from build123d import *

# Parameters (mm, degrees)
F0_W     = 152.4
F0_H     = 25.4
F1_DEPTH = 50.8
F2_D     = 4.2
F2_DEPTH = 18
F2_TIP   = 1.2618073
F3_D     = 5
F3_DEPTH = 20
F3_TIP   = 1.5021515476
F4_D     = 6.8
F4_DEPTH = 25
F4_TIP   = 2.0429261047
F5_D     = 8.5
F5_DEPTH = 25
F5_TIP   = 2.5536576309
F6_D     = 10.3
F6_DEPTH = 40
F6_TIP   = 3.094432188
F7_R     = 2


with BuildPart() as f1:
    # F0 (on Top) → F1 (new body)
    with BuildSketch(Plane.XY):
        with Locations((22.0912756948, 0)):
            Rectangle(F0_W, F0_H)
    extrude(amount=-F1_DEPTH)

    # F2
    with Locations(Plane.XY):
        with Locations((-28.7087243052, 0)):
            Hole(F2_D / 2, depth=F2_DEPTH)
            with Locations((0, 0, -(F2_DEPTH + F2_TIP / 2))):  # 118° drill point
                Cone(0, F2_D / 2, F2_TIP, mode=Mode.SUBTRACT)

    # F3
    with Locations(Plane.XY):
        with Locations((-3.3087243052, 0)):
            Hole(F3_D / 2, depth=F3_DEPTH)
            with Locations((0, 0, -(F3_DEPTH + F3_TIP / 2))):  # 118° drill point
                Cone(0, F3_D / 2, F3_TIP, mode=Mode.SUBTRACT)

    # F4
    with Locations(Plane.XY):
        with Locations((22.0912756948, 0)):
            Hole(F4_D / 2, depth=F4_DEPTH)
            with Locations((0, 0, -(F4_DEPTH + F4_TIP / 2))):  # 118° drill point
                Cone(0, F4_D / 2, F4_TIP, mode=Mode.SUBTRACT)

    # F5
    with Locations(Plane.XY):
        with Locations((47.4912756948, 0)):
            Hole(F5_D / 2, depth=F5_DEPTH)
            with Locations((0, 0, -(F5_DEPTH + F5_TIP / 2))):  # 118° drill point
                Cone(0, F5_D / 2, F5_TIP, mode=Mode.SUBTRACT)

    # F6
    with Locations(Plane.XY):
        with Locations((72.8912756948, 0)):
            Hole(F6_D / 2, depth=F6_DEPTH)
            with Locations((0, 0, -(F6_DEPTH + F6_TIP / 2))):  # 118° drill point
                Cone(0, F6_D / 2, F6_TIP, mode=Mode.SUBTRACT)

    # F7
    f7_edges = [f1.edges().sort_by_distance(p)[0] for p in [
        (22.091276, -12.7, 0),
        (98.291276, 0, 0),
        (22.091276, 12.7, 0),
        (-54.108724, 0, 0),
        (98.291276, 12.7, -25.4),
        (98.291276, -12.7, -25.4),
        (-54.108724, 12.7, -25.4),
        (-54.108724, -12.7, -25.4),
    ]]
    fillet(f7_edges, radius=F7_R)


solid = f1.part
Design review of the part built by this model. Coordinates are the model's own, in mm. A direction names the side the tool comes from. Coordinates: 2 decimals unless noted, no trailing zeros. Write each loop counter-clockwise with the first axis right and the second up, starting at its lowest first coordinate (ties: lowest second). Pieces come first, ordered by that corner, then holes. Notation, with made-up numbers: (59.5, 2.25) -> (112.5, 2.25) arc R12 cw to (112.5, 20.25) -> close; hole circle Ø1 at (10.5, 3.25). An arc over 180 degrees is marked (long way). Write each question's results on one line, items separated by ' | '. Start each with the question number.
(1) Tool access review of faces 4 (the face through (50.6, 2.9, -12.7)), 5 (the face through (21, -5, 0)): name each direction out of +Z, -Z, +X, -X, +Y, -Y from which nothing blocks a thin tool from reaching the whole face with its end or side.
(2) Clearance check with a flat-ended pin moving along its axis: P1, Ø3.5, axis at x = -28.71, y = 0, coming from the +Z side. State where the tip first meets the part, or that it passes through.
(3) Take a section at A-A on z = -32.5. Write out the cut boundary in (x, y), and give its area (3 significant figures).
(4) The part is to be moulded in two halves that separate along Y. For faces 1 (the face through (-54.109, 0, -26)), 2 (the face through (78.036, 0.226, -20.28)), 3 (the face through (21, -12.7, -26)), say which applies: pulls with the +Y half, pulls with the -Y half, needs draft (parallel to the pull), parting line crosses it, or undercut.
(5) For line 1 along X through (y, z) = (0, -16); line 2 along X through (y, z) = (-0.25, -28.5); line 3 along X through (y, z) = (0, -20.5), list the stretches that pass through material, from the lowest coordinate up. Write a range as from..to.
Results found:
1) face 4: +Z | face 5: +Z, +X, -X, +Y, -Y
2) P1: stops at z = -18.21
3) outline: (-54.11, -10.7) arc R2 ccw to (-52.11, -12.7) -> (96.29, -12.7) arc R2 ccw to (98.29, -10.7) -> (98.29, 10.7) arc R2 ccw to (96.29, 12.7) -> (-52.11, 12.7) arc R2 ccw to (-54.11, 10.7) -> close; hole circle Ø10.3 at (72.89, 0) | area: 3,780 mm2
4) face 1: needs draft | face 2: undercut | face 3: pulls with the -Y half
5) line 1: x = -54.11..-30.81, -26.61..-5.81, -0.81..18.69, 25.49..43.24, 51.74..67.74, 78.04..98.29 | line 2: x = -54.11..67.75, 78.04..98.29 | line 3: x = -54.11..-4.98, -1.64..18.69, 25.49..43.24, 51.74..67.74, 78.04..98.29
